Autodesk Inventor part; units mm, degrees
ref_plane "YZ Plane" through (0, 0, 0) normal (1, 0, 0) x (0, 1, 0)
ref_plane "XZ Plane" through (0, 0, 0) normal (0, 1, 0) x (-1, 0, 0)
ref_plane "XY Plane" through (0, 0, 0) normal (0, 0, 1) x (1, 0, 0)
sketch "Sketch1" plane through (0, 0, 0) normal (0, 0, 1) x (1, 0, 0)
  line L0 (0, 0) -> (30, 0)
  line L1 (30, 0) -> (30, 30)
  line L2 (30, 30) -> (0, 30)
  line L3 (0, 30) -> (0, 0)
  dimension "d0" = 30
  dimension "d1" = 30
extrude "Extrusion1" add sketch "Sketch1" along normal blind 3
sketch "Sketch2" plane through (0, 0, 3) normal (0, 0, 1) x (1, 0, 0)
  line L0 (30, 3.6) -> (2.6, 3.6)
  line L1 (2.6, 3.6) -> (2.6, 29)
  line L2 (2.6, 29) -> (30, 29)
  line L3 (30, 29) -> (30, 3.6)
  line L4 (0, 0) -> (30, 0)
  line L5 (30, 0) -> (30, 30)
  dimension "d4" = 27.4
  dimension "d5" = 25.4
  dimension "d36" = 3.6
extrude "Extrusion2" cut sketch "Sketch2" against normal blind 0.5
sketch "Sketch3" plane through (0, 0, 3) normal (0, 0, 1) x (1, 0, 0)
  line L0 (30, 30) -> (0, 30)
  line L1 (0, 30) -> (0, 0)
  line L2 (28, 30) -> (0, 30)
  line L3 (0, 30) -> (0, 29)
  line L4 (0, 29) -> (28, 29)
  line L5 (28, 29) -> (28, 30)
  line L6 (30, 29) -> (30, 30)
  line L7 (0, 0) -> (30, 0)
  line L8 (28, 0) -> (0, 0)
  line L9 (0, 0) -> (0, 1)
  line L10 (0, 1) -> (28, 1)
  line L11 (28, 1) -> (28, 0)
  line L12 (30, 0) -> (30, 3.6)
  dimension "d8" = 1
  dimension "d9" = 2
  dimension "d10" = 1
  dimension "d11" = 2
extrude "Extrusion3" cut sketch "Sketch3" against normal through all
sketch "Sketch4" plane through (0, 0, 3) normal (0, 0, 1) x (1, 0, 0)
  line L0 (30, 29) -> (30, 30)
  line L1 (30, 30) -> (-0.4, 30)
  line L2 (-0.4, 30) -> (-0.4, 31)
  line L3 (-0.4, 31) -> (30, 31)
  line L4 (30, 31) -> (30, 30)
  line L5 (30, 0) -> (-0.4, 0)
  line L6 (-0.4, 0) -> (-0.4, -1)
  line L7 (-0.4, -1) -> (30, -1)
  line L8 (30, -1) -> (30, 0)
  line L9 (2, 31) -> (3, 31)
  line L10 (3, 31) -> (3, 31.6)
  line L11 (3, 31.6) -> (2, 31.6)
  line L12 (2, 31.6) -> (2, 31)
  line L13 (2, -1) -> (3, -1)
  line L14 (3, -1) -> (3, -1.6)
  line L15 (3, -1.6) -> (2, -1.6)
  line L16 (2, -1.6) -> (2, -1)
  line L17 (0, 29) -> (0, 1)
  point P0 (0, 0)
  dimension "d14" = 30.4
  dimension "d15" = 1
  dimension "d17" = 1
  dimension "d20" = 1
  dimension "d21" = 0.6
  dimension "d26" = 1
  dimension "d27" = 0.6
  dimension "d35" = 2
extrude "Extrusion4" add sketch "Sketch4" against normal blind 3
chamfer "Chamfer1" distance 1 angle 45 4 edges at (30, 31, 1.5) (30, -1, 1.5) (28, 1, 1.5) (28, 30, 1.5)
chamfer "Chamfer2" distance 1 angle 45 2 edges at (29.0005, 31, 1.5) (29.0005, -1, 1.5)
chamfer "Chamfer3" distance 1 angle 45 2 edges at (0, 29, 1.5) (0, 1, 1.5)
chamfer "Chamfer4" distance 1 angle 45 2 edges at (1, 29, 1.5) (1, 1, 1.5)
properties part number "TA10" material "ABS Plastic"
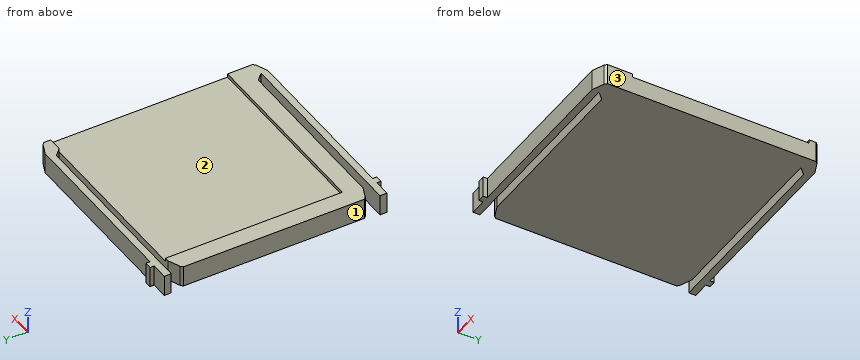
Design review of the part built by this model. Coordinates are the model's own, in mm. Face numbers are marked on the shaded views. Coordinates: 2 decimals unless noted, no trailing zeros. Order: outer loops, then holes, each group sorted by start corner. A loop starts at its lowest first (then second) coordinate and runs counter-clockwise, first axis right, second up. Notation, with made-up numbers: (41, -30.5) -> (71, -30.5) arc R25 ccw to (71, -8.5) -> close; hole circle Ø4 at (10, -15.5). An arc over 180 degrees is marked (long way). Use one line per item in the form item = value. Start each with the question number.
(1) Add section C-C on y = 26. State the section outline as (x, z) points.
(2) For probe 1 along Y at (x, z) = (20.5, 0.75); probe 2 along Y at (x, z) = (6, 2.7); probe 3 along Z at (x, y) = (11.5, 12), list the stretches that pass through material, from the lowest coordinate up.
(3) The part is to be moulded in two halves that separate along Y. For the marked faces 1, 2 and 3, say which applies: +Y half, -Y half, draft (parallel to the pull), parting line (faces both ways), or undercut.
(4) Insertion check: pin 1 (0.9 mm diameter, centred on x = 15, z = 2, fed in from -Y); pin 2 (0.6 mm diameter, centred on y = 18, z = 3, fed in from +X); pin 3 (10 mm diameter, centred on x = 22.5, y = 12.5, fed in from +Z). Each pin has a flat end and moves straight along its axis. Give the tip position at first contact, or say it passes through.
(5) Add section A-A on x = 25.5. State the section outline as (y, z) points.
Answer block:
q1.outline = (0, 0) -> (30, 0) -> (30, 2.5) -> (2.6, 2.5) -> (2.6, 3) -> (0, 3) -> close
q2.probe_1 = -1 to 0, 1 to 29, 30 to 31
q2.probe_2 = -1 to 0, 1 to 3.6, 30 to 31
q2.probe_3 = 0 to 2.5
q3.face_1 = undercut
q3.face_2 = undercut
q3.face_3 = draft
q4.pin_1 = -1
q4.pin_2 = 2.6
q4.pin_3 = 2.5
q5.outline = (-1, 0) -> (0, 0) -> (0, 3) -> (-1, 3) -> close; (1, 0) -> (29, 0) -> (29, 2.5) -> (3.6, 2.5) -> (3.6, 3) -> (1, 3) -> close; (30, 0) -> (31, 0) -> (31, 3) -> (30, 3) -> close
